The figure shows three views and two pictorial views of one solid part (mm, origin at its lowest corner). Answer the questions. A direction names the side the tool comes from. Coordinates: 2 decimals unless noted, no trailing zeros. Write each loop counter-clockwise with the first axis right and the second up, starting at its lowest first coordinate (ties: lowest second). Pieces come first, ordered by that corner, then holes. Notation, with made-up numbers: M 54,36 L 63,36 A38 cw 63,74 Z; hole C 5.5,73 d3. An arc over 180 degrees is marked long. Write item = value, one per line.
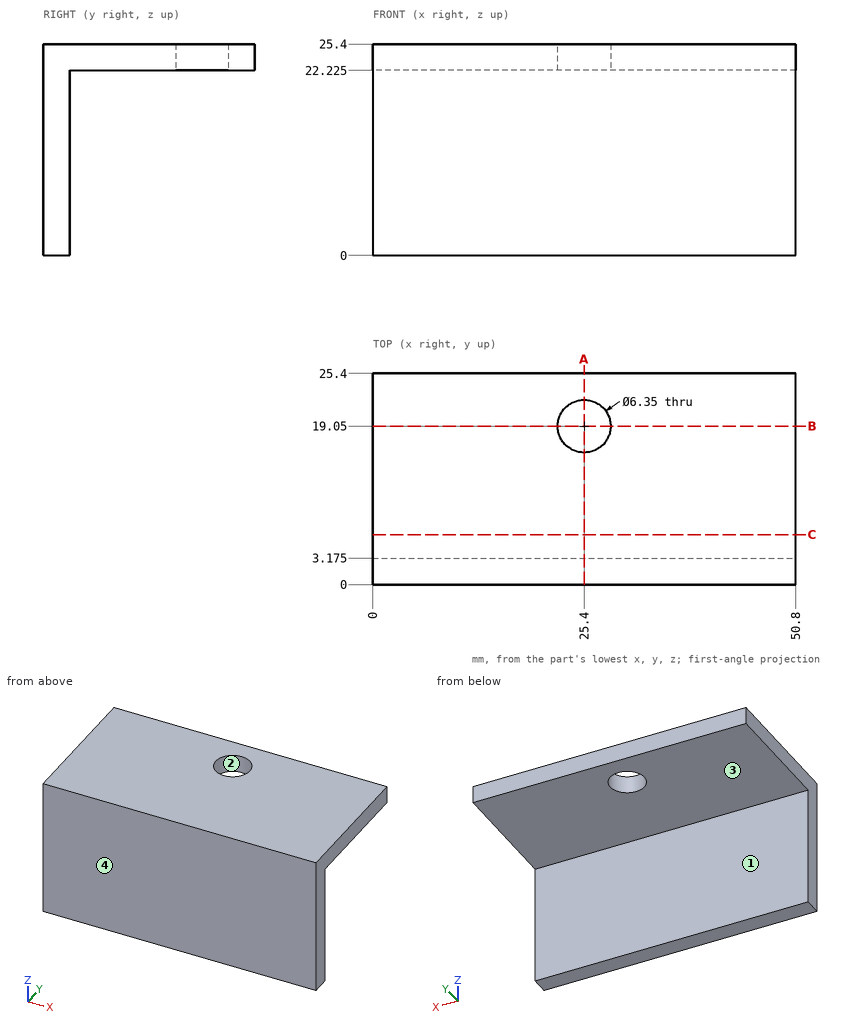
Item 1: Consider line 1 along Y through (x, z) = (25.4, 22.9) (3 decimals); line 2 along Y through (x, z) = (13.5, 17.75) (3 decimals); line 3 along Z through (x, y) = (30, 16.5) (3 decimals). Determine where each line is inside the solid, lowest interval first. Write a range as from..to.
Worked answers:
line_1 = 0..15.875, 22.225..25.4
line_2 = 0..3.175
line_3 = 22.225..25.4
Item 2: Which of the six approach directions +Z, -Z, +X, -X, +Y, -Y give full straight-line access (tool end or side, diameter ignored) to the marked faces 3 and 4?
Worked answers:
face_3 = -Z, +X, -X, +Y
face_4 = +Z, -Z, +X, -X, -Y
Item 3: Find section C-C (y = 6). Determine the outline of the cut face in (x, z) (3 decimals).
Worked answers:
outline = M 0,22.225 L 50.8,22.225 L 50.8,25.4 L 0,25.4 Z
Item 4: Find section B-B (y = 19.05). Determine the outline of the cut face in (x, z) (3 decimals), and give its area (3 significant figures).
Worked answers:
outline = M 0,22.225 L 22.225,22.225 L 22.225,25.4 L 0,25.4 Z; M 28.575,22.225 L 50.8,22.225 L 50.8,25.4 L 28.575,25.4 Z
area = 141 mm²
Item 5: For a pull along X with two mould halves and no side action, classify the marked faces 1 and 2 as released by +X, released by -X, zero draft, split by the parting line, or undercut.
Worked answers:
face_1 = zero draft
face_2 = undercut
Item 6: Find section A-A (x = 25.4). Determine the outline of the cut face in (y, z) (3 decimals), and give its area (3 significant figures).
Worked answers:
outline = M 0,0 L 3.175,0 L 3.175,22.225 L 15.875,22.225 L 15.875,25.4 L 0,25.4 Z; M 22.225,22.225 L 25.4,22.225 L 25.4,25.4 L 22.225,25.4 Z
area = 131 mm²
Item 7: Flat-ended cylindrical pins translate along their axes: pin 1 (4 mm diameter, centred on x = 36, y = 9, fed in from -Z) (3 decimals); pin 2 (12 mm diameter, centred on x = 29, z = 12.5, fed in from +Y) (3 decimals). Find the tip coordinate at first contact, or state that the pin passes through.
Worked answers:
pin_1 = 22.225
pin_2 = 3.175
